Verification items for the finished model (mm, model axes). Face numbers are marked on the shaded views. Round coordinates to 2 decimals unless told otherwise and drop trailing zeros. Order: outer loops, then holes, each group sorted by start corner. A loop starts at its lowest first (then second) coordinate and runs counter-clockwise, first axis right, second up. Notation, with made-up numbers: (8, 23) -> (52, 23) arc R15 ccw to (52, 28) -> close; hole circle Ø9 at (27.25, 87.25). An arc over 180 degrees is marked (long way). Return JSON: item names as keys, results as strings. Group by question number.
1) Section check A-A on z = 40.5. Enter the section's corners in (x, y).
2) Scan lines: L1, parallel to Y at x = -8.5, z = 5.5; L2, parallel to X at y = 17.5, z = 21.5; L3, parallel to Y at x = -29.5, z = 36.5. Record each from-to range of solid material in increasing order.
3) Section check B-B on z = 26. Enter the section's corners in (x, y), plus the area to 3 significant figures.
4) Draft check along Y on the marked faces 1, 2 and 3. Enter one of: pulls with the +Y half, pulls with the -Y half, needs draft (parallel to the pull), parting line crosses it, or undercut.
5) Depth check by flat-ended pin: pin 1 (2 mm diameter, centred on x = -28.5, y = 9, fed in from +Z); pin 2 (6 mm diameter, centred on x = 1, y = -14.5, fed in from -Z); pin 3 (4 mm diameter, centred on y = 26, z = 20.5, fed in from -X); pin 4 (4 mm diameter, centred on x = 0, z = 36, fed in from -Y). Enter the tip coordinate at first touch or a pass-through.
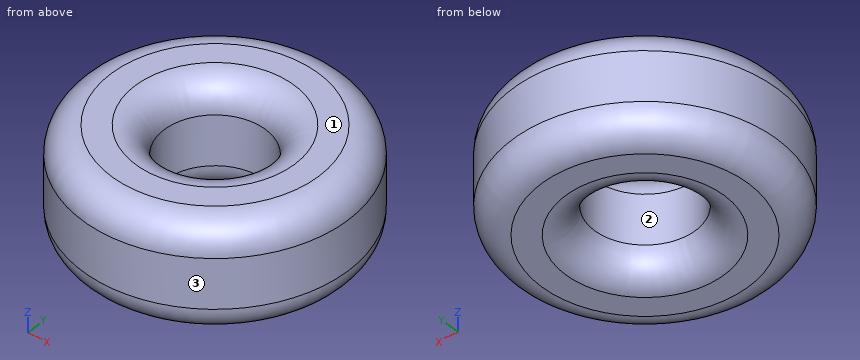
```python
from build123d import *

# Parameters (mm, degrees)
SKETCH2_R           = 55
SKETCH2_R_2         = 21
BOSS_EXTRUDE1_DEPTH = 44.5
FILLET1_R           = 12


with BuildPart() as part:
    # Sketch2 → Boss-Extrude1 (new body)
    with BuildSketch(Plane.XY):
        with Locations((-9.780925239, 3.803880586)):
            Circle(SKETCH2_R)
        with Locations((-9.780925239, 3.803880586)):
            Circle(SKETCH2_R_2, mode=Mode.SUBTRACT)
    extrude(amount=BOSS_EXTRUDE1_DEPTH)

    # Fillet1
    fillet1_edges = [part.edges().sort_by_distance(p)[0] for p in [
        (-64.780925239, 3.803880586, 0),
        (-64.780925239, 3.803880586, 44.5),
        (-30.780925239, 3.803880586, 0),
        (-30.780925239, 3.803880586, 44.5),
    ]]
    fillet(fillet1_edges, radius=FILLET1_R)


solid = part.part
```
Check result:
{
 "1": {"outline": "circle Ø103.89 at (-9.78, 3.8); hole circle Ø48.11 at (-9.78, 3.8)"},
 "2": {"L1": "-49.27 to -19.07, 26.68 to 56.88", "L2": "-63.05 to -25.7, 6.14 to 43.49", "L3": "-46.8 to -5.22, 12.83 to 54.41"},
 "3": {"outline": "circle Ø110 at (-9.78, 3.8); hole circle Ø42 at (-9.78, 3.8)", "area": "8,120 mm^2"},
 "4": {"face 1": "needs draft", "face 2": "undercut", "face 3": "parting line crosses it"},
 "5": {"pin 1": "through", "pin 2": "z = 3.8", "pin 3": "x = -60.94", "pin 4": "y = -50.37"}
}
